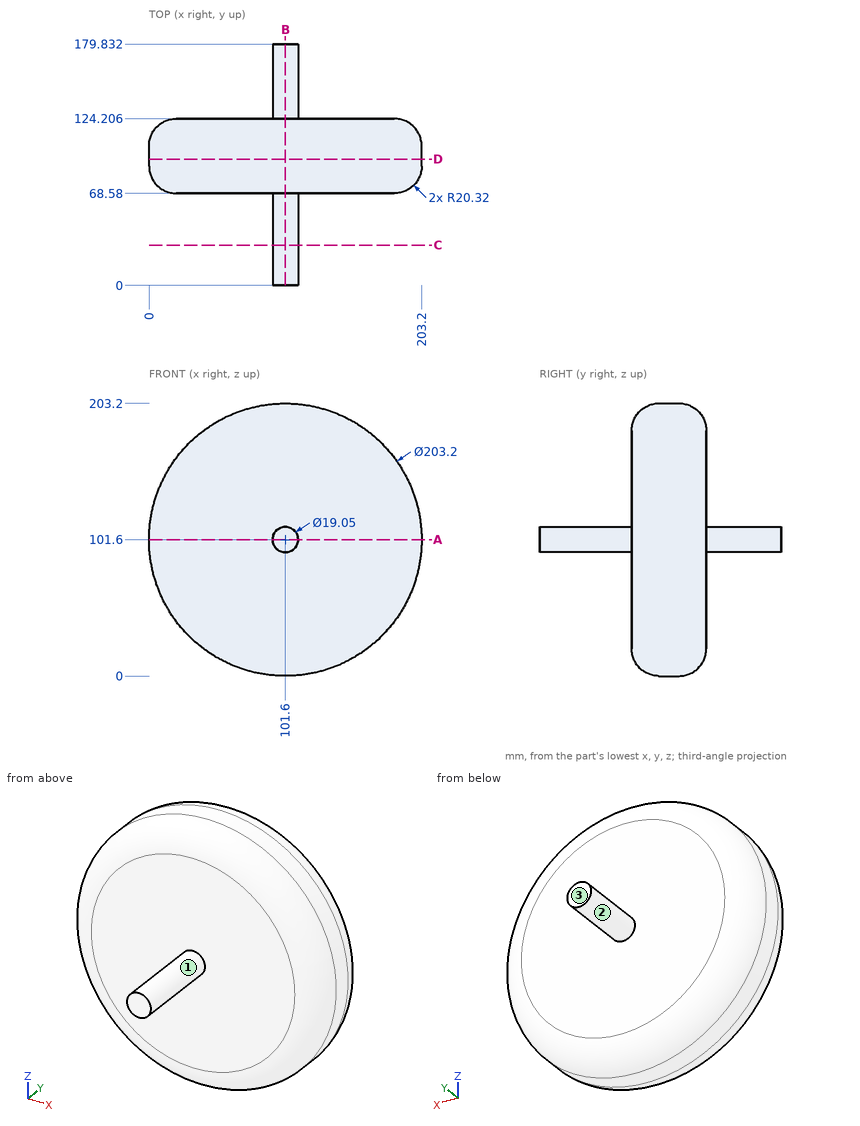
Design review of the part shown in the three views and the two pictorial views. Dimensions are in mm from the part's minimum x, y and z. A direction names the side the tool comes from. Coordinates: 2 decimals unless noted, no trailing zeros. Write each loop counter-clockwise with the first axis right and the second up, starting at its lowest first coordinate (ties: lowest second). Pieces come first, ordered by that corner, then holes.
(1) Wall thickness on probe 1 along Y at (x, z) = (155, 158.5); probe 2 along Z at (x, y) = (101.5, 52.5); probe 3 along X at (y, z) = (106.5, 90.5): over which ranges is each line inside the solid? List them lowest first.
(2) Add section D-D on y = 94. Give the boundary of the cut face in (x, z).
(3) For pin 1 Ø3 at (x, z) = (72, 157) entering from +Y; pin 2 Ø10 at (y, z) = (125, 41.5) entering from +X; pin 3 Ø12 at (x, z) = (179.5, 80) entering from -Y, all flat-tipped, find the tip position at first contact; note any pin that passes through.
(4) Add section B-B on x = 101.6. Give the boundary of the cut face in (y, z) (3 decimals), then the cut area to 3 significant figures.
(5) Tool access review of the marked faces 1, 2 and 3: name each direction out of +Z, -Z, +X, -X, +Y, -Y from which nothing blocks a thin tool from reaching the whole face with its end or side.
(6) Add section A-A on z = 101.6. Give the boundary of the cut face in (x, y) (3 decimals).
(7) Add section C-C on y = 30. Give the boundary of the cut face in (x, z) (3 decimals).
Answer sheet:
1. probe 1: y = 68.58 to 124.21
1. probe 2: z = 92.08 to 111.12
1. probe 3: x = 0.78 to 202.42
2. outline: circle Ø203.2 at (101.6, 101.6)
3. pin 1: stops at y = 124.21
3. pin 2: stops at x = 174.34
3. pin 3: stops at y = 68.58
4. outline: (0, 92.075) - (68.58, 92.075) - (68.58, 20.32) arc R20.32 ccw to (88.9, 0) - (103.886, 0) arc R20.32 ccw to (124.206, 20.32) - (124.206, 92.075) - (179.832, 92.075) - (179.832, 111.125) - (124.206, 111.125) - (124.206, 182.88) arc R20.32 ccw to (103.886, 203.2) - (88.9, 203.2) arc R20.32 ccw to (68.58, 182.88) - (68.58, 111.125) - (0, 111.125) - close
4. area: 13,300 mm2
5. face 1: -Y
5. face 2: +Y
5. face 3: +Z, -Z, +X, -X, +Y
6. outline: (0, 88.9) arc R20.32 ccw to (20.32, 68.58) - (92.075, 68.58) - (92.075, 0) - (111.125, 0) - (111.125, 68.58) - (182.88, 68.58) arc R20.32 ccw to (203.2, 88.9) - (203.2, 103.886) arc R20.32 ccw to (182.88, 124.206) - (111.125, 124.206) - (111.125, 179.832) - (92.075, 179.832) - (92.075, 124.206) - (20.32, 124.206) arc R20.32 ccw to (0, 103.886) - close
7. outline: circle Ø19.05 at (101.6, 101.6)
